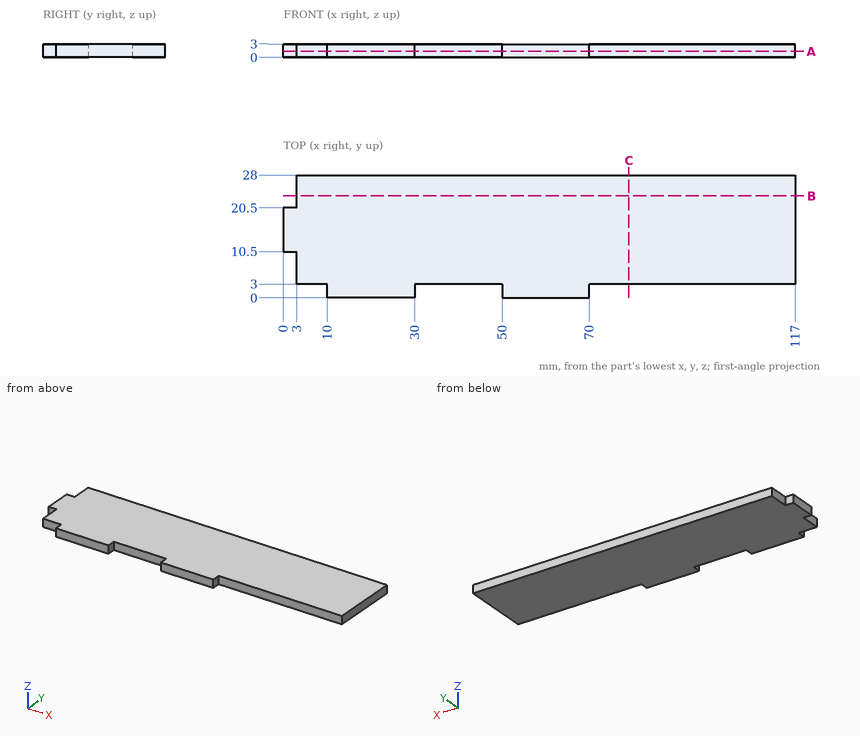
The drawing under review shows one solid part. Ordinate dimensions are in mm from its lowest x, y, z. Give positions to 0.01 mm unless a question says otherwise; leave off trailing zeros. Loops run counter-clockwise (first coordinate to the right, second up) from the corner with the lowest first, then second, coordinate; pieces in that order, holes last. Notation, with made-up numbers: M 20,-18.5 L 67,-18.5 A28 cw 67,18.5 Z; hole C -3,57.5 d4. An arc over 180 degrees is marked long. Return JSON: item names as keys, results as strings. Group by question number.
Item 1: We need section B-B (y = 23.25). Give the boundary of the cut face in (x, z).
Item 2: Insertion check: pin 1 Ø0.9 at (x, z) = (86, 1) entering from -Y; pin 2 Ø1.5 at (y, z) = (1, 1.5) entering from -X; pin 3 Ø0.9 at (y, z) = (1.5, 1.5) entering from +X. Each pin has a flat end and moves straight along its axis. Give the tip position at first contact, or say it passes through.
Item 3: For probe 1 along X at (y, z) = (23.75, 1.8); probe 2 along Y at (x, z) = (100, 2.95); probe 3 along X at (y, z) = (1.5, 1.55), list the stretches that pass through material, from the lowest coordinate up.
Item 4: We need section C-C (x = 79). Give the boundary of the cut face in (y, z), and give its area (3 significant figures).
Item 5: We need section A-A (z = 1.3). Give the boundary of the cut face in (x, y).
Output:
{
 "1": {"outline": "M 3,0 L 117,0 L 117,3 L 3,3 Z"},
 "2": {"pin 1": "stops at y = 3", "pin 2": "stops at x = 10", "pin 3": "stops at x = 70"},
 "3": {"probe 1": "x = 3 to 117", "probe 2": "y = 3 to 28", "probe 3": "x = 10 to 30, 50 to 70"},
 "4": {"outline": "M 3,0 L 28,0 L 28,3 L 3,3 Z", "area": "75.0 mm^2"},
 "5": {"outline": "M 0,10.5 L 3,10.5 L 3,3 L 10,3 L 10,0 L 30,0 L 30,3 L 50,3 L 50,0 L 70,0 L 70,3 L 117,3 L 117,28 L 3,28 L 3,20.5 L 0,20.5 Z"}
}
